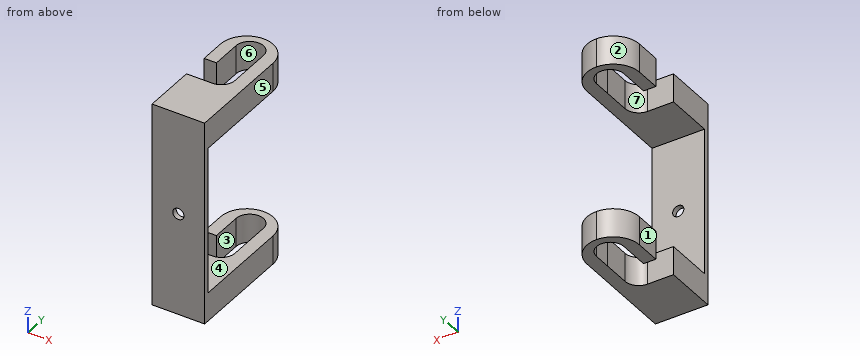
Autodesk Inventor part; units mm, degrees
ref_plane "YZ Plane" through (0, 0, 0) normal (1, 0, 0) x (0, 1, 0)
ref_plane "XZ Plane" through (0, 0, 0) normal (0, 1, 0) x (-1, 0, 0)
ref_plane "XY Plane" through (0, 0, 0) normal (0, 0, 1) x (1, 0, 0)
sketch "Sketch1" plane through (0, 0, 0) normal (0, 1, 0) x (-1, 0, 0)
  line L0 (10, 67.88) -> (-10, 67.88)
  line L1 (-10, 67.88) -> (-10, -10)
  line L2 (-10, -10) -> (10, -10)
  line L3 (10, -10) -> (10, 67.88)
  point P0 (0, 0)
  dimension "d0" = 20
  dimension "d1" = 77.88
extrude "Extrusion1" add sketch "Sketch1" along normal blind 2
sketch "Sketch2" plane through (0, 2, 0) normal (0, 1, 0) x (1, 0, 0)
  line L0 (-10, -67.88) -> (10, -67.88)
  line L1 (0, -67.88) -> (-6.35, -67.88)
  line L2 (-6.35, -56.98) -> (6.35, -56.98)
  line L3 (6.35, -67.88) -> (0, -67.88)
  line L4 (10, 10) -> (-10, 10)
  line L5 (-6.35, -0.9) -> (6.35, -0.9)
  line L6 (-6.35, 10) -> (6.35, 10)
  line L7 (-6.35, -67.88) -> (-10, -67.88)
  line L8 (-10, 10) -> (-10, -67.88)
  line L9 (-10, -56.98) -> (-6.35, -56.98)
  line L10 (6.35, -67.88) -> (10, -67.88)
  line L11 (10, -67.88) -> (10, 10)
  line L12 (10, -56.98) -> (6.35, -56.98)
  line L13 (6.35, -0.9) -> (10, -0.9)
  line L14 (10, 10) -> (6.35, 10)
  line L15 (10, -0.9) -> (10, 10)
  line L16 (10, -67.88) -> (10, -56.98)
  line L17 (-10, -67.88) -> (-10, -56.98)
  line L18 (-6.35, -0.9) -> (-10, -0.9)
  line L19 (-10, -0.9) -> (-10, 10)
  line L20 (-10, 10) -> (-6.35, 10)
  point P0 (0, 0)
  dimension "d4" = 6.35
  dimension "d5" = 10.9
  dimension "d6" = 12.7
  dimension "d7" = 10.9
extrude "Extrusion2" add sketch "Sketch2" along normal blind 48.3354 contours L8 L9 L2 L12 L11 L0 | L8 L4 L11 L13 L5 L18
sketch "Sketch9" plane through (-10, 0, 67.88) normal (0, 0, 1) x (1, 0, 0)
  arc A0 (15.084, 42.3223) -> (4.684, 42.3223) centre (9.884, 42.3223) ccw
  line L0 (15.084, 35.9247) -> (15.084, 42.3223)
  line L1 (4.684, 41.1247) -> (4.684, 42.3223)
  arc A1 (15.084, 42.3223) -> (4.684, 42.3223) centre (9.884, 42.3223) ccw
  line L2 (4.684, 42.3223) -> (4.684, 35.9247)
  line L3 (9.8827, 20.3222) -> (-0.0013, 20.3222)
  line L4 (-0.0013, 30.726) -> (-0.0013, 20.3222)
  line L5 (4.684, 35.9247) -> (4.684, 30.726)
  line L6 (15.084, 35.9247) -> (15.0853, 25.5254)
  arc A2 (15.084, 35.9247) -> (15.084, 35.9251) centre (9.884, 35.9243) ccw
  line L7 (4.684, 30.726) -> (-0.0013, 30.726)
  arc A3 (9.8827, 20.3222) -> (15.0853, 25.5254) centre (9.8827, 25.5248) ccw
  point P0 (10, 0)
fillet "Fillet4" radius 10 4 edges at (10, 50.3354, 62.43) (-10, 50.3354, 62.43) (-10, 50.3354, -4.55) (10, 50.3354, -4.55)
sketch "Sketch10" plane through (0, 2, 0) normal (0, 1, 0) x (1, 0, 0)
  line L0 (10, -67.88) -> (-10, -67.88)
  line L1 (-10, 10) -> (10, 10)
  line L2 (10, -56.98) -> (10, -0.9)
  line L3 (-10, -0.9) -> (-10, -56.98)
  line L4 (10, -28.94) -> (-10, -28.94)
  circle A0 centre (0, -28.94) radius 2.125
  point P0 (0, 0)
  dimension "d53" = 77.88
  dimension "d54" = 4.25
extrude "Extrusion10" cut sketch "Sketch10" against normal blind 2
extrude "Extrusion11" cut sketch "Sketch9" against normal through all
properties part number "6 Backet Adjustment"
Design review of the part built by this model. Coordinates are the model's own, in mm. Face numbers are marked on the shaded views. A direction names the side the tool comes from. Give positions to 0.01 mm unless a question says otherwise; leave off trailing zeros. Loops run counter-clockwise (first coordinate to the right, second up) from the corner with the lowest first, then second, coordinate; pieces in that order, holes last. Notation, with made-up numbers: (-26.75, 37.25) -> (5.25, 37.25) arc R34 ccw to (5.25, 76.25) -> close; hole circle Ø5 at (10, 7.5). An arc over 180 degrees is marked (long way). Write each question's results on one line, items separated by ' | '.
Q1. Machinability: for the marked faces 4, 5, 6 and 7, which of the approach directions +Z, -Z, +X, -X, +Y, -Y give a long, thin tool a straight path to every point of the face, cutting with its end or side? Answer none if there is none.
Reply:
face 4: +X, -X, +Y | face 5: +Z, -Z, +X, +Y, -Y | face 6: +Z, -Z | face 7: +Z, -Z, -X
Q2. Wall thickness on L1, parallel to Z at x = 0, y = 1.35 (3 decimals); L2, parallel to Z at x = -1.5, y = 10; L3, parallel to Y at x = -5.5, z = 29: over which ranges is each line inside the solid? List them lowest first.
Reply:
L1: z = -10 to 26.815, 31.065 to 67.88 | L2: z = -10 to 0.9, 56.98 to 67.88 | L3: y = 0 to 2
Q3. Take a section at C-C, the plane x = -7.5. Write out the cut boundary in (y, z), plus the area to 3 significant figures.
Reply:
outline: (0, -10) -> (20.32, -10) -> (20.32, 0.9) -> (2, 0.9) -> (2, 56.98) -> (20.32, 56.98) -> (20.32, 67.88) -> (0, 67.88) -> close; (30.73, -10) -> (46.95, -10) -> (46.95, 0.9) -> (30.73, 0.9) -> close; (30.73, 56.98) -> (46.95, 56.98) -> (46.95, 67.88) -> (30.73, 67.88) -> close | area: 909 mm²
Q4. Take a section at D-D, the plane y = 8. Write out the cut boundary in (x, z), plus the area to 3 significant figures.
Reply:
outline: (-10, -10) -> (10, -10) -> (10, 0.9) -> (-10, 0.9) -> close; (-10, 56.98) -> (10, 56.98) -> (10, 67.88) -> (-10, 67.88) -> close | area: 436 mm²
Q5. Take a section at A-A, the plane z = 28.94. Write out the cut boundary in (x, y) (3 decimals), plus the area to 3 significant figures.
Reply:
outline: (-10, 0) -> (-2.125, 0) -> (-2.125, 2) -> (-10, 2) -> close; (2.125, 0) -> (10, 0) -> (10, 2) -> (2.125, 2) -> close | area: 31.5 mm²
Q6. The part is to be moulded in two halves that separate along Y. For the marked faces 1, 2 and 3, say which applies: +Y half, -Y half, draft (parallel to the pull), parting line (faces both ways), or undercut.
Reply:
face 1: draft | face 2: +Y half | face 3: undercut
Q7. For pin 1 Ø3 at (x, z) = (-5.5, -4.5) entering from +Y; pin 2 Ø1.5 at (x, z) = (5.5, 36) entering from +Y; pin 3 Ø3 at (x, z) = (-4.5, 61.5) entering from +Y, all flat-tipped, find the tip position at first contact; note any pin that passes through.
Reply:
pin 1: stops at y = 49.5 | pin 2: stops at y = 2 | pin 3: stops at y = 49.87
Q8. Take a section at B-B, the plane y = 38. Write out the cut boundary in (x, z).
Reply:
outline: (-10, -10) -> (-5.32, -10) -> (-5.32, 0.9) -> (-10, 0.9) -> close; (-10, 56.98) -> (-5.32, 56.98) -> (-5.32, 67.88) -> (-10, 67.88) -> close; (5.08, -10) -> (10, -10) -> (10, 0.9) -> (5.08, 0.9) -> close; (5.08, 56.98) -> (10, 56.98) -> (10, 67.88) -> (5.08, 67.88) -> close
